The model under review builds one solid part; all positions refer to its coordinate system, in mm. A direction names the side the tool comes from. Round coordinates to 2 decimals unless told otherwise and drop trailing zeros. Order: outer loops, then holes, each group sorted by start corner. A loop starts at its lowest first (then second) coordinate and runs counter-clockwise, first axis right, second up. Notation, with made-up numbers: (23.5, 86.25) -> (40.5, 86.25) arc R21 ccw to (40.5, 111.25) -> close; hole circle Ø1 at (37, -20.75). An arc over 180 degrees is marked (long way). Return JSON: item names as keys, results as strings. Group by question number.
from build123d import *

# Parameters (mm, degrees)
MOTOR_START                     = -30
MOTOR_HOLDER_DEPTH              = 50
SKETCH11_R                      = 5
SCREW_HOLES_DEPTH               = 109.397416943
FILLET1_R                       = 10
BOSS_EXTRUDE4_DEPTH             = 10
BOSS_EXTRUDE4_DEPTH_BACK        = 10
SKETCH14_R                      = 18.090252651
BOSS_EXTRUDE5_REACH             = 122.52
SKETCH17_R                      = 10
BOSS_EXTRUDE5_DIRECTION_2_DEPTH = 1
BOSS_EXTRUDE6_DEPTH             = 10
BOSS_EXTRUDE6_DEPTH_BACK        = 44
SKETCH18_R                      = 20
SKETCH18_R_2                    = 10


with BuildPart() as part:
    # Sketch1 → motor holder (new body)
    with BuildSketch(Plane.XY.offset(MOTOR_START)):
        with BuildLine():
            Line((-35, 35), (-25, 35))
            ThreePointArc((-25, 35), (0, 10), (25, 35))
            Line((25, 35), (35, 35))
            ThreePointArc((35, 35), (0, 0), (-35, 35))
        make_face()
    motor_holder = extrude(amount=MOTOR_HOLDER_DEPTH)

    # Mirror1: motor holder across plane
    add(motor_holder.mirror(Plane(origin=(25, 35, -30), x_dir=(0, 0, 1), z_dir=(0, -1, 0))))

    # Sketch10 → bearing holder (revolve)
    with BuildSketch(Plane(origin=(0, 0, 0), x_dir=(0, 0, -1), z_dir=(1, 0, 0)), mode=Mode.PRIVATE) as bearing_holder_sk:
        Polygon((-20, 5), (-20, -10), (0, -10), (0, -15), (10, -15), (10, 5), align=None)
    revolve(bearing_holder_sk.sketch.rotate(Axis((0, -40, 67.918923046), (0, 0, -1)), 90), axis=Axis((0, -40, 67.918923046), (0, 0, -1)))

    # Sketch11 → screw holes (cut, through all)
    with BuildSketch(Plane.XY.offset(20)):
        with Locations((0, -77.5)):
            Circle(SKETCH11_R)
        with Locations((-26.516504294, -66.516504294)):
            Circle(SKETCH11_R)
        with Locations((-37.5, -40)):
            Circle(SKETCH11_R)
        with Locations((-26.516504294, -13.483495706)):
            Circle(SKETCH11_R)
        with Locations((0, -2.5)):
            Circle(SKETCH11_R)
        with Locations((26.516504294, -13.483495706)):
            Circle(SKETCH11_R)
        with Locations((37.5, -40)):
            Circle(SKETCH11_R)
        with Locations((26.516504294, -66.516504294)):
            Circle(SKETCH11_R)
    extrude(amount=-SCREW_HOLES_DEPTH, mode=Mode.SUBTRACT)

    # Fillet1
    fillet1_edges = [part.edges().sort_by_distance(p)[0] for p in [
        (13.795127964, 2.833333333, 5),
        (-13.795127964, 2.833333333, 5),
    ]]
    fillet(fillet1_edges, radius=FILLET1_R)

    # Sketch14 → Boss-Extrude4 (add, two sides: drawn at the far end of the back side and taken through both)
    with BuildSketch(Plane(origin=(35, 0, 0), x_dir=(0, 0, -1), z_dir=(1, 0, 0)).offset(-BOSS_EXTRUDE4_DEPTH_BACK)):
        with Locations((0, 35)):
            Circle(SKETCH14_R)
    extrude(amount=BOSS_EXTRUDE4_DEPTH + BOSS_EXTRUDE4_DEPTH_BACK)

    # Sketch17 → Boss-Extrude5 (add, up to next)
    with BuildSketch(Plane.ZY.offset(35), mode=Mode.PRIVATE) as boss_extrude5_sk1:
        with Locations(Location((5.095876685, 0, 0), (0, 0, 202.728422598))):
            Circle(SKETCH17_R)
    boss_extrude5_tool1 = extrude(boss_extrude5_sk1.sketch, amount=-BOSS_EXTRUDE5_REACH, mode=Mode.PRIVATE) - part.part
    add(boss_extrude5_tool1.solids().sort_by_distance((-35, 0, 5.095877))[0])

    # Sketch17 → Boss-Extrude5 direction 2 (add)
    with BuildSketch(Plane.ZY.offset(35)):
        with Locations(Location((5.095876685, 0, 0), (0, 0, 202.728422598))):
            Circle(SKETCH17_R)
    extrude(amount=BOSS_EXTRUDE5_DIRECTION_2_DEPTH)

    # Sketch18 → Boss-Extrude6 (add, two sides: drawn at the far end of the back side and taken through both)
    with BuildSketch(Plane(origin=(0, 0, -4.904123315), x_dir=(-1, 0, 0), z_dir=(0, 0, -1)).offset(-BOSS_EXTRUDE6_DEPTH_BACK)):
        with Locations((53.320508076, 0)):
            Circle(SKETCH18_R)
        with Locations((53.320508076, 0)):
            Circle(SKETCH18_R_2, mode=Mode.SUBTRACT)
    extrude(amount=BOSS_EXTRUDE6_DEPTH + BOSS_EXTRUDE6_DEPTH_BACK)


solid = part.part
Item 1: Wall thickness on line 1 along X through (y, z) = (35, -15); line 2 along Y through (x, z) = (37, 1); line 3 along Y through (x, z) = (-36, 5): over which ranges is each line inside the solid? List them lowest first.
Item 2: Insertion check: pin 1 Ø10 at (x, z) = (-12, -17) entering from +Y; pin 2 Ø16 at (x, y) = (0, -2.5) entering from +Z; pin 3 Ø1.5 at (x, z) = (-28, -5) entering from -Y. Each pin has a flat end and moves straight along its axis. Give the tip position at first contact, or say it passes through.
Item 3: Consider section B-B on x = -56. State the section outline as (y, z) points, plus the area to 3 significant figures.
Item 4: For faces 4 (the face through (-29.28, 9.84, 3.32)), 5 (the face through (-6.503, -10.713, 9.86)), 6 (the face through (-1.08, -82.38, 5.21)), 7 (the face through (39.047, 35.795, 18.073)), 8 (the face through (-48.6, 9.2, 39.096)), list the 3-axis set-ups (+Z, -Z, +X, -X, +Y, -Y) from which the entire face can be reached by the end or side of a thin tool; tool diameter is ignored.
Item 5: Consider section C-C on x = 12.5. State the section outline as (y, z) points, plus the area to 3 significant figures.
Item 6: Consider section A-A on y = -40. State the section outline as (x, z) points.
Item 7: The part is to be moulded in two halves that separate along X. For faces 1 (the face through (45, 35, 0)), 2 (the face through (-7, -65, 0)), 3 (the face through (24, 43, -30)), say which applies: +X half, -X half, draft (parallel to the pull), parting line (faces both ways), or undercut.
Item 8: Consider section D-D on z = 31.5. State the section outline as (x, y) points, plus the area to 3 significant figures.
Values:
{
 "1": {"line 1": "-35 to -25, 25 to 45", "line 2": "-65.61 to -44.97, -35.03 to -14.39, 16.94 to 53.06", "line 3": "-67 to -44.77, -35.23 to -13, -10 to 10"},
 "2": {"pin 1": "y = 69.29", "pin 2": "z = 20", "pin 3": "y = -75.81"},
 "3": {"outline": "(-19.82, -14.9) -> (-9.63, -14.9) -> (-9.63, 39.1) -> (-19.82, 39.1) -> close; (9.63, -14.9) -> (19.82, -14.9) -> (19.82, 39.1) -> (9.63, 39.1) -> close", "area": "1,100 mm^2"},
 "4": {"face 4": "none", "face 5": "+Z", "face 6": "+Z, -Z", "face 7": "+X", "face 8": "+Z, +X, -X, +Y, -Y"},
 "5": {"outline": "(-83.23, -10) -> (-61.65, -10) -> (-61.65, 0) -> (-67.27, 0) -> (-67.27, 20) -> (-83.23, 20) -> close; (-18.35, -10) -> (2.31, -10) -> (2.31, -30) -> (13.35, -30) -> (13.35, 20) -> (-12.73, 20) -> (-12.73, 0) -> (-18.35, 0) -> close; (56.65, -30) -> (67.69, -30) -> (67.69, 20) -> (56.65, 20) -> close", "area": "2,150 mm^2"},
 "6": {"outline": "(-45, -10) -> (-42.5, -10) -> (-42.5, 20) -> (-45, 20) -> close; (-32.5, -10) -> (-25, -10) -> (-25, 0) -> (-30, 0) -> (-30, 20) -> (-32.5, 20) -> close; (25, -10) -> (32.5, -10) -> (32.5, 20) -> (30, 20) -> (30, 0) -> (25, 0) -> close; (42.5, -10) -> (45, -10) -> (45, 20) -> (42.5, 20) -> close"},
 "7": {"face 1": "+X half", "face 2": "undercut", "face 3": "draft"},
 "8": {"outline": "circle Ø40 at (-53.32, 0); hole circle Ø20 at (-53.32, 0)", "area": "942 mm^2"}
}
